For this review, take the finished solid that the model builds, in its own axes (mm). A direction names the side the tool comes from. Give positions to 0.01 mm unless a question says otherwise; leave off trailing zeros. Loops run counter-clockwise (first coordinate to the right, second up) from the corner with the lowest first, then second, coordinate; pieces in that order, holes last. Notation, with made-up numbers: (-12.75, 19) -> (-5.75, 19) arc R23 ccw to (-5.75, 28) -> close; hole circle Ø1 at (53, -1). An arc over 180 degrees is marked (long way). Answer as CSV lines item,"result". Start each with the question number.
Item 1: Add section A-A on y = 0. State the section outline as (x, z) points (3 decimals).
Item 2: For L1, parallel to Y at x = 0, z = 17 (3 decimals); L2, parallel to Z at x = 2, y = 22; L3, parallel to X at y = 15, z = -11.5, list the stretches that pass through material, from the lowest coordinate up. Write a range as from..to.
Item 3: The part is to be moulded in two halves that separate along Z. For faces 5 (the face through (0.037, 5.715, 0.178)), 6 (the face through (0, 13, 19.05)), 7 (the face through (-0.21, -5.71, -15.83)), 8 (the face through (0, 13, -19.05)), say which applies: +Z half, -Z half, draft (parallel to the pull), parting line (faces both ways), or undercut.
Item 4: Clearance check with flat-ended pins moving along their axes: P1, Ø5.5, axis at x = -2, y = 26.5, coming from the +Z side; P2, Ø3, axis at y = 6.5, z = 4, coming from the +X side; P3, Ø12, axis at y = 16, z = 4, coming from the -X side; P4, Ø5.5, axis at x = 0, y = 25.4, coming from the -Z side. State where each tip first meets the part, or that it passes through.
Item 5: Machinability: for faces 1 (the face through (-0.037, 19.685, -0.178)), 2 (the face through (-2.54, 13, 0)), 3 (the face through (0.21, 31.11, -15.83)), 4 (the face through (2.54, 13, 0)), which of the approach directions +Z, -Z, +X, -X, +Y, -Y give a long, thin tool a straight path to every point of the face, cutting with its end or side? Answer none if there is none.
Item 6: Add section D-D on x = -5. State the section outline as (y, z) points.
Item 7: Add section B-B on x = 0. State the section outline as (y, z) points (3 decimals), plus the area to 3 significant figures.
Item 8: Add section C-C on z = -15.5. State the section outline as (x, y) points (3 decimals), plus the area to 3 significant figures.
```python
from build123d import *

# Parameters (mm, degrees)
SKETCH1_R           = 3.175
BOSS_EXTRUDE1_DEPTH = 19.05
SKETCH1_3_R         = 5.715
SKETCH1_3_R_2       = 3.175
CUT_EXTRUDE2_DEPTH  = 12.7


with BuildPart() as part:
    # Sketch1 → Boss-Extrude1 (new body, symmetric)
    with BuildSketch(Plane.XY):
        with BuildLine():
            ThreePointArc((2.54, 20.28046633), (0, 31.115), (-2.54, 20.28046633))
            Line((-2.54, 20.28046633), (-2.54, 5.11953367))
            ThreePointArc((-2.54, 5.11953367), (0, -5.715), (2.54, 5.11953367))
            Line((2.54, 5.11953367), (2.54, 20.28046633))
        make_face()
        with Locations((0, 25.4)):
            Circle(SKETCH1_R, mode=Mode.SUBTRACT)
        Circle(SKETCH1_R, mode=Mode.SUBTRACT)
    extrude(amount=BOSS_EXTRUDE1_DEPTH, both=True)

    # Sketch1_3 → Cut-Extrude2 (cut, symmetric)
    with BuildSketch(Plane.XY):
        with Locations((0, 25.4)):
            Circle(SKETCH1_3_R)
        with Locations((0, 25.4)):
            Circle(SKETCH1_3_R_2, mode=Mode.SUBTRACT)
        Circle(SKETCH1_3_R)
        Circle(SKETCH1_3_R_2, mode=Mode.SUBTRACT)
    extrude(amount=CUT_EXTRUDE2_DEPTH, both=True, mode=Mode.SUBTRACT)


solid = part.part
```
Computed values:
1,outline,"(-5.715, -19.05) -> (-3.175, -19.05) -> (-3.175, -12.7) -> (-5.715, -12.7) -> close; (-5.715, 12.7) -> (-3.175, 12.7) -> (-3.175, 19.05) -> (-5.715, 19.05) -> close; (3.175, -19.05) -> (5.715, -19.05) -> (5.715, -12.7) -> (3.175, -12.7) -> close; (3.175, 12.7) -> (5.715, 12.7) -> (5.715, 19.05) -> (3.175, 19.05) -> close"
2,L1,"-5.715..-3.175, 3.175..22.225, 28.575..31.115"
2,L2,"-19.05..-12.7, 12.7..19.05"
2,L3,"-2.54..2.54"
3,face 5,"undercut"
3,face 6,"+Z half"
3,face 7,"draft"
3,face 8,"-Z half"
4,P1,"z = 19.05"
4,P2,"x = 2.54"
4,P3,"x = -2.54"
4,P4,"through"
5,face 1,"+Y"
5,face 2,"+Z, -Z, -X"
5,face 3,"+Z, -Z"
5,face 4,"+Z, -Z, +X"
6,outline,"(-2.77, -19.05) -> (2.77, -19.05) -> (2.77, -12.7) -> (-2.77, -12.7) -> close; (-2.77, 12.7) -> (2.77, 12.7) -> (2.77, 19.05) -> (-2.77, 19.05) -> close; (22.63, -19.05) -> (28.17, -19.05) -> (28.17, -12.7) -> (22.63, -12.7) -> close; (22.63, 12.7) -> (28.17, 12.7) -> (28.17, 19.05) -> (22.63, 19.05) -> close"
7,outline,"(-5.715, -19.05) -> (-3.175, -19.05) -> (-3.175, -12.7) -> (-5.715, -12.7) -> close; (-5.715, 12.7) -> (-3.175, 12.7) -> (-3.175, 19.05) -> (-5.715, 19.05) -> close; (3.175, -19.05) -> (22.225, -19.05) -> (22.225, -12.7) -> (19.685, -12.7) -> (19.685, 12.7) -> (22.225, 12.7) -> (22.225, 19.05) -> (3.175, 19.05) -> (3.175, 12.7) -> (5.715, 12.7) -> (5.715, -12.7) -> (3.175, -12.7) -> close; (28.575, -19.05) -> (31.115, -19.05) -> (31.115, -12.7) -> (28.575, -12.7) -> close; (28.575, 12.7) -> (31.115, 12.7) -> (31.115, 19.05) -> (28.575, 19.05) -> close"
7,area,"661 mm²"
8,outline,"(-2.54, 5.12) arc R5.715 ccw (long way) to (2.54, 5.12) -> (2.54, 20.28) arc R5.715 ccw (long way) to (-2.54, 20.28) -> close; hole circle Ø6.35 at (0, 0); hole circle Ø6.35 at (0, 25.4)"
8,area,"215 mm²"
